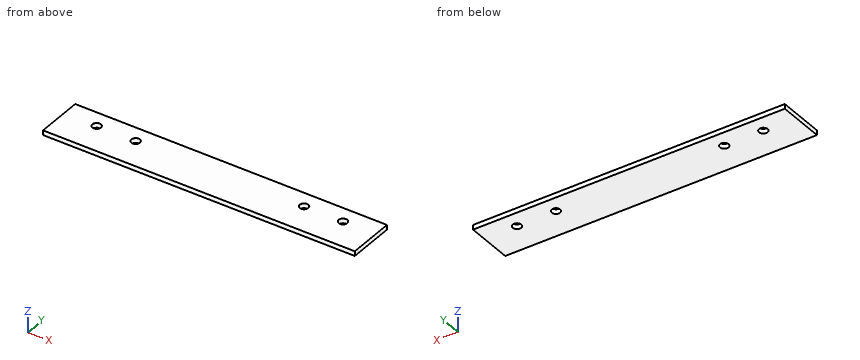
from build123d import *

# Parameters (mm, degrees)
SKETCH1_W                      = 200
SKETCH1_H                      = 30
BOSS_EXTRUDE1_DEPTH            = 1.5
M5_CLEARANCE_HOLE1_D           = 5.5
M5_CLEARANCE_HOLE1_CSINK_D     = 5.55
M5_CLEARANCE_HOLE1_CSINK_ANGLE = 90


with BuildPart() as part:
    # Sketch1 → Boss-Extrude1 (new, symmetric)
    with BuildSketch(Plane.XY):
        Rectangle(SKETCH1_W, SKETCH1_H)
    extrude(amount=BOSS_EXTRUDE1_DEPTH, both=True)

    # M5 Clearance Hole1 (through all)
    with Locations(Plane.XY.offset(1.5)):
        with Locations((54, 4.5), (-79, 4.5), (-54, 4.5), (79, 4.5)):
            CounterSinkHole(M5_CLEARANCE_HOLE1_D / 2, M5_CLEARANCE_HOLE1_CSINK_D / 2, counter_sink_angle=M5_CLEARANCE_HOLE1_CSINK_ANGLE)


solid = part.part
Read the model definition and answer for the solid it produces. Units are mm, in the model's axes. Coordinates: 2 decimals unless noted, no trailing zeros. Loops run counter-clockwise (first coordinate to the right, second up) from the corner with the lowest first, then second, coordinate; pieces in that order, holes last. Notation, with made-up numbers: (-20, -17.5) - (-8, -17.5) arc R28 ccw to (-8, 10.5) - close; hole circle Ø11 at (53.5, 47.25). An arc over 180 degrees is marked (long way). Answer in a Markdown table with one row per item.
Q1. Find section C-C on y = 4.5. Write down the section's boundary in (x, z) (3 decimals), plus the area to 3 significant figures.
Here are the results:
| item | result |
|---|---|
| outline | (-100, -1.5) - (-81.75, -1.5) - (-81.75, 1.475) - (-81.775, 1.5) - (-100, 1.5) - close; (-76.25, -1.5) - (-56.75, -1.5) - (-56.75, 1.475) - (-56.775, 1.5) - (-76.225, 1.5) - (-76.25, 1.475) - close; (-51.25, -1.5) - (51.25, -1.5) - (51.25, 1.475) - (51.225, 1.5) - (-51.225, 1.5) - (-51.25, 1.475) - close; (56.75, -1.5) - (76.25, -1.5) - (76.25, 1.475) - (76.225, 1.5) - (56.775, 1.5) - (56.75, 1.475) - close; (81.75, -1.5) - (100, -1.5) - (100, 1.5) - (81.775, 1.5) - (81.75, 1.475) - close |
| area | 534 mm^2 |
Q2. Find section B-B on x = -79. Write down the section's boundary in (y, z) (3 decimals), plus the area to 3 significant figures.
Here are the results:
| item | result |
|---|---|
| outline | (-15, -1.5) - (1.75, -1.5) - (1.75, 1.475) - (1.725, 1.5) - (-15, 1.5) - close; (7.25, -1.5) - (15, -1.5) - (15, 1.5) - (7.275, 1.5) - (7.25, 1.475) - close |
| area | 73.5 mm^2 |
Q3. Find section A-A on z = -0.1. Write down the section's boundary in (x, y).
Here are the results:
| item | result |
|---|---|
| outline | (-100, -15) - (100, -15) - (100, 15) - (-100, 15) - close; hole circle Ø5.5 at (-79, 4.5); hole circle Ø5.5 at (-54, 4.5); hole circle Ø5.5 at (54, 4.5); hole circle Ø5.5 at (79, 4.5) |
Q4. Straight lines are drawn through the part: line 1 along X through (y, z) = (4.5, 0.1); line 2 along Y through (x, z) = (-79, 0.15); line 3 along Y through (x, z) = (52, -0.15). For each, find the intervals that lie inside material, in ascending order. Write a range as [from, to].
Here are the results:
| item | result |
|---|---|
| line 1 | x = [-100, -81.75], [-76.25, -56.75], [-51.25, 51.25], [56.75, 76.25], [81.75, 100] |
| line 2 | y = [-15, 1.75], [7.25, 15] |
| line 3 | y = [-15, 2.61], [6.39, 15] |
